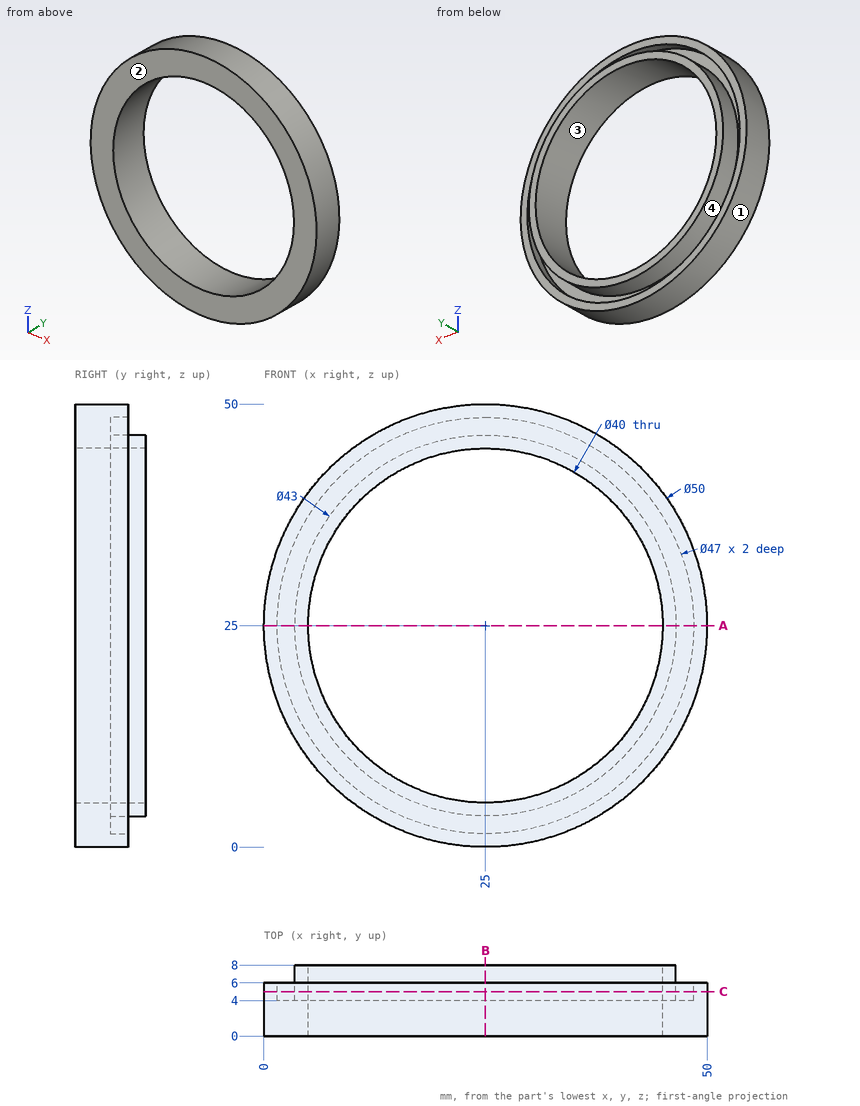
Verification items for this drawing (mm, ordinates from the low corner). Coordinates: 2 decimals unless noted, no trailing zeros. Write each loop counter-clockwise with the first axis right and the second up, starting at its lowest first coordinate (ties: lowest second). Pieces come first, ordered by that corner, then holes. Notation, with made-up numbers: M 85.25,83.25 L 144.25,83.25 A18 ccw 144.25,113.25 Z; hole C -35,-20 d1. An arc over 180 degrees is marked long. One line per item, written item: value. Start each with the question number.
(1) Sectioned sample at B-B, the plane x = 25. Enter the section's corners in (y, z).
(2) Release check for a two-part mould opening along Z. For the marked faces 1, 2, 3 and 4 record: released by +Z, released by -Z, zero draft, split by the parting line, or undercut.
(3) Depth check by flat-ended pin: pin 1 (1 mm diameter, centred on x = 5.5, y = 1, fed in from +Z); pin 2 (12 mm diameter, centred on x = 14.5, z = 33.5, fed in from -Y). Enter the tip coordinate at first touch or a pass-through.
(4) Scan lines: line 1 along Z through (x, y) = (11.5, 5); line 2 along X through (y, z) = (2.5, 24.5) (3 decimals); line 3 along Z through (x, y) = (39, 5). Record each from-to range of solid material in increasing order. Write a range as [from, to].
(5) Sectioned sample at A-A, the plane z = 25. Enter the section's corners in (x, y), and give its area (3 significant figures).
(6) Sectioned sample at C-C, the plane y = 5. Enter the section's corners in (x, z).
Filled sheet:
1. outline: M 0,0 L 6,0 L 6,1.5 L 4,1.5 L 4,3.5 L 8,3.5 L 8,5 L 0,5 Z; M 0,45 L 8,45 L 8,46.5 L 4,46.5 L 4,48.5 L 6,48.5 L 6,50 L 0,50 Z
2. face 1: split by the parting line
2. face 2: zero draft
2. face 3: undercut
2. face 4: undercut
3. pin 1: z = 41.25
3. pin 2: through
4. line 1: [3.96, 5.76], [8.27, 10.24], [39.76, 41.73], [44.24, 46.04]
4. line 2: [0.005, 5.006], [44.994, 49.995]
4. line 3: [4.29, 6.13], [8.68, 10.72], [39.28, 41.32], [43.87, 45.71]
5. outline: M 0,0 L 5,0 L 5,8 L 3.5,8 L 3.5,4 L 1.5,4 L 1.5,6 L 0,6 Z; M 45,0 L 50,0 L 50,6 L 48.5,6 L 48.5,4 L 46.5,4 L 46.5,8 L 45,8 Z
5. area: 58.0 mm²
6. outline: C 25,25 d50; C 25,25 d43; hole C 25,25 d47; hole C 25,25 d40
